The model under review builds one solid part; all positions refer to its coordinate system, in mm. Face numbers are marked on the shaded views. A direction names the side the tool comes from. Round coordinates to 2 decimals unless told otherwise and drop trailing zeros. Loops run counter-clockwise (first coordinate to the right, second up) from the corner with the lowest first, then second, coordinate; pieces in that order, holes last. Notation, with made-up numbers: (51, -38) -> (85, -38) arc R25 cw to (85, -9) -> close; hole circle Ø2 at (-18.75, 65.25). An arc over 180 degrees is marked (long way). Use a Markdown table: item, result. Add a question column.
1) Consider section B-B on z = 0. Give the boundary of the cut face in (x, y) (3 decimals).
2) Mouldability with a two-part tool opening along X and no side actions: class the marked faces 3, 4, 5 and 6 as released by +X, released by -X, zero draft, split by the parting line, or undercut.
3) Consider section D-D on y = -42. Give the boundary of the cut face in (x, z), plus the area to 3 significant figures.
4) Wall thickness on probe 1 along Z at (x, y) = (0, 7.5); probe 2 along X at (y, z) = (10, 0.5) (3 decimals); probe 3 along X at (y, z) = (-17, 0) (3 decimals): over which ranges is each line inside the solid? List them lowest first.
5) For the marked faces 1 and 2, list the 3-axis set-ups (+Z, -Z, +X, -X, +Y, -Y) from which the entire face can be reached by the end or side of a thin tool; tool diameter is ignored.
6) Consider section A-A on x = 0. Give the boundary of the cut face in (y, z).
7) Consider section C-C on y = 5. Give the boundary of the cut face in (x, z) (3 decimals).
8) Insertion check: pin 1 (5 mm diameter, centred on x = -29, z = -31.5, fed in from -Y); pin 2 (1.5 mm diameter, centred on y = -36, z = -28.5, fed in from +X); pin 3 (8 mm diameter, centred on x = -37, y = -33.5, fed in from +Z); pin 4 (4 mm diameter, centred on y = -39, z = 24.5, fed in from -X). Each pin has a flat end and moves straight along its axis. Give the tip position at first contact, or say it passes through.
from build123d import *

# Parameters (mm, degrees)
F0_W      = 110.49001
F0_H      = 81.642858
F1_DEPTH  = 25.4
F1_FACE_W = 110.49001
F1_FACE_H = 81.642858
F2_DEPTH  = 25.4
F4_R      = 31.45223
F5_DEPTH  = 47.498
F3_R      = 21.081854
F6_DEPTH  = 117.856
F7_R      = 20.698965
F8_DEPTH  = 81.534


with BuildPart() as f1:
    # F0 (on Front) → F1 (new body)
    with BuildSketch(Plane.XZ):
        Rectangle(F0_W, F0_H)
    extrude(amount=F1_DEPTH)

    # F1_face (on face) → F2 (join)
    with BuildSketch(Plane(origin=(0, 0, 0), x_dir=(1, 0, 0), z_dir=(0, 1, 0))):
        Rectangle(F1_FACE_W, F1_FACE_H)
    extrude(amount=F2_DEPTH)

    # F4 (on Front) → F5 (join)
    with BuildSketch(Plane.XZ):
        Circle(F4_R)
    extrude(amount=F5_DEPTH)

    # F3 (on Front) → F6 (cut)
    with BuildSketch(Plane.XZ):
        Circle(F3_R)
    extrude(amount=F6_DEPTH, mode=Mode.SUBTRACT)

    # F7 (on Front) → F8 (cut)
    with BuildSketch(Plane.XZ):
        Circle(F7_R)
    extrude(amount=-F8_DEPTH, mode=Mode.SUBTRACT)


solid = f1.part
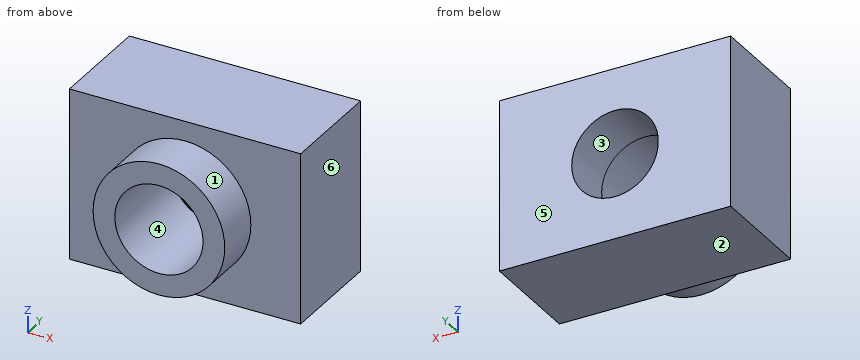
Result set:
| question | item | result |
|---|---|---|
| 1 | outline | (-55.245, -25.4) -> (-31.452, -25.4) -> (-31.452, -47.498) -> (-21.082, -47.498) -> (-21.082, 0) -> (-20.699, 0) -> (-20.699, 25.4) -> (-55.245, 25.4) -> close; (20.699, 0) -> (21.082, 0) -> (21.082, -47.498) -> (31.452, -47.498) -> (31.452, -25.4) -> (55.245, -25.4) -> (55.245, 25.4) -> (20.699, 25.4) -> close |
| 2 | face 3 | undercut |
| 2 | face 4 | undercut |
| 2 | face 5 | zero draft |
| 2 | face 6 | released by +X |
| 3 | outline | circle Ø62.9 at (0, 0); hole circle Ø42.16 at (0, 0) |
| 3 | area | 1,710 mm2 |
| 4 | probe 1 | -40.82 to -20.7, 20.7 to 40.82 |
| 4 | probe 2 | -55.245 to -20.693, 20.693 to 55.245 |
| 4 | probe 3 | -55.245 to -21.082, 21.082 to 55.245 |
| 5 | face 1 | -Y |
| 5 | face 2 | -Z, +X, -X, +Y, -Y |
| 6 | outline | (-47.5, -31.45) -> (-25.4, -31.45) -> (-25.4, -40.82) -> (25.4, -40.82) -> (25.4, -20.7) -> (0, -20.7) -> (0, -21.08) -> (-47.5, -21.08) -> close; (-47.5, 21.08) -> (0, 21.08) -> (0, 20.7) -> (25.4, 20.7) -> (25.4, 40.82) -> (-25.4, 40.82) -> (-25.4, 31.45) -> (-47.5, 31.45) -> close |
| 7 | outline | (-55.245, -40.821) -> (55.245, -40.821) -> (55.245, 40.821) -> (-55.245, 40.821) -> close; hole circle Ø41.398 at (0, 0) |
| 8 | pin 1 | y = -25.4 |
| 8 | pin 2 | x = 14.8 |
| 8 | pin 3 | through |
| 8 | pin 4 | x = -21.98 |
